Geometry check sheet. Reference: drawing and pictorial views, mm from the part's lowest x, y, z. Give positions to 0.01 mm unless a question says otherwise; leave off trailing zeros. Loops run counter-clockwise (first coordinate to the right, second up) from the corner with the lowest first, then second, coordinate; pieces in that order, holes last. Notation, with made-up numbers: (-35.5, 69) - (-8.5, 69) arc R17 ccw to (-8.5, 89) - close; hole circle Ø5 at (70.5, -35.75). An arc over 180 degrees is marked (long way). Answer in a Markdown table with one row per item. Add a question column.
(1) Sectioned sample at C-C on x = 80.5. Enter the section's corners in (y, z) (1 decimal).
(2) Sectioned sample at B-B on z = 1.85. State how many separate pieces and enclosed holes the cut face has, then the cut area to 3 significant figures.
(3) Thickness scan on L1, parallel to X at y = 27.5, z = 1.65 (1 decimal); L2, parallel to X at y = 80, z = 1; L3, parallel to Y at x = 82.5, z = 2.2 (1 decimal). Record the ranges inside material, lowest first.
(4) Go/stop test with a flat-tipped pin: P1, Ø1, axis at x = 71, y = 61, coming from the -Z side. Record where the tip stops, or that it passes through.
(5) Sectioned sample at A-A on x = 61. Enter the section's corners in (y, z) (1 decimal).
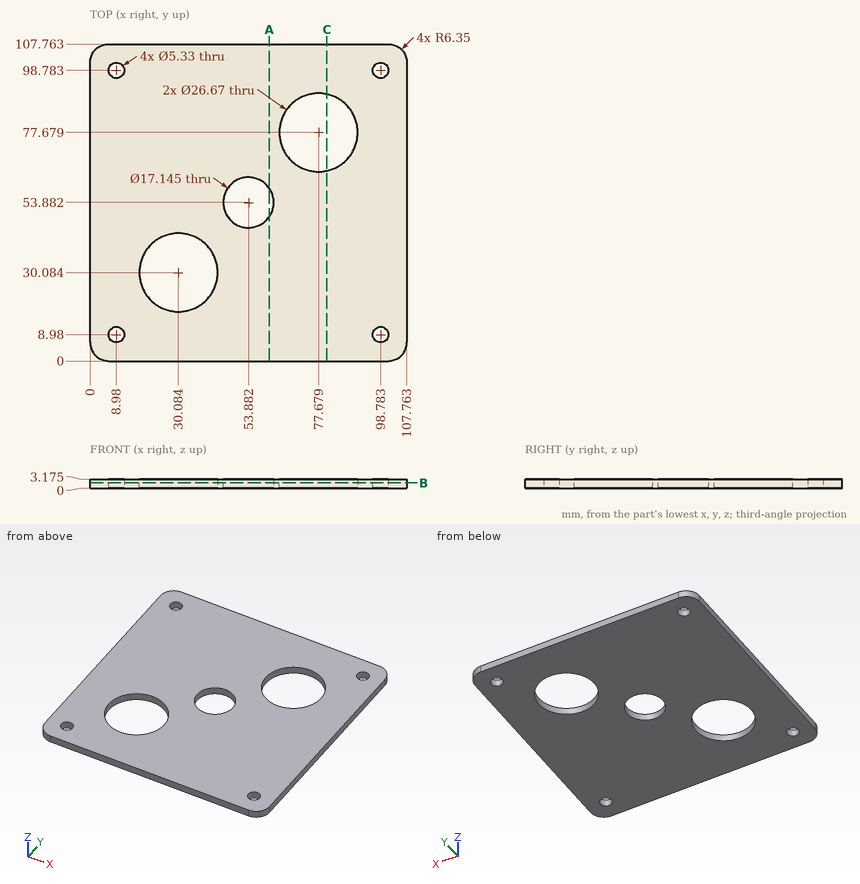
Reply:
| question | item | result |
|---|---|---|
| 1 | outline | (0, 0) - (64.6, 0) - (64.6, 3.2) - (0, 3.2) - close; (90.7, 0) - (107.8, 0) - (107.8, 3.2) - (90.7, 3.2) - close |
| 2 | separate pieces | 1 |
| 2 | enclosed holes | 7 |
| 2 | area | 10,100 mm^2 |
| 3 | L1 | 0 to 17, 43.2 to 107.8 |
| 3 | L2 | 0 to 64.55, 90.81 to 107.76 |
| 3 | L3 | 0 to 65.2, 90.1 to 107.8 |
| 4 | P1 | z = 0 |
| 5 | outline | (0, 0) - (49.1, 0) - (49.1, 3.2) - (0, 3.2) - close; (58.7, 0) - (107.8, 0) - (107.8, 3.2) - (58.7, 3.2) - close |
